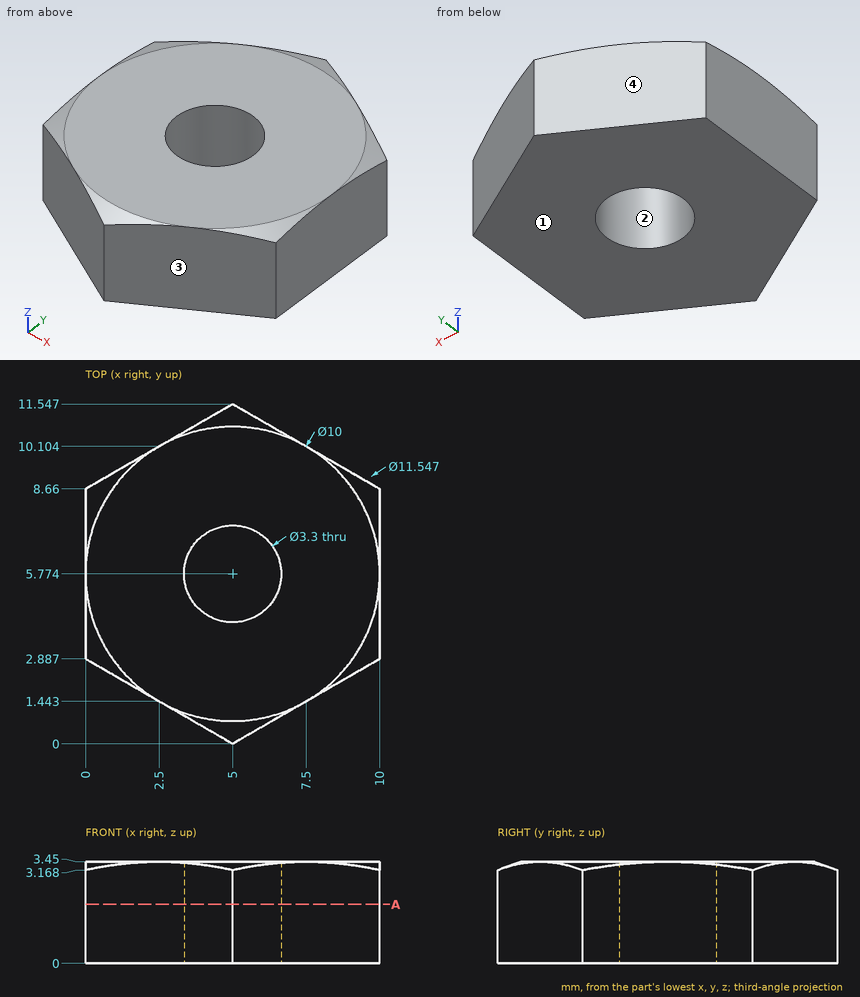
Design review of the part shown in the three views and the two pictorial views. Dimensions are in mm from the part's minimum x, y and z. Round coordinates to 2 decimals unless told otherwise and drop trailing zeros. Order: outer loops, then holes, each group sorted by start corner. A loop starts at its lowest first (then second) coordinate and runs counter-clockwise, first axis right, second up.
Item 1: To check wall thickness, follow probe 1 along X at (y, z) = (5.75, 2.5); probe 2 along X at (y, z) = (6.5, 1.1); probe 3 along Y at (x, z) = (4, 3.05) (1 decimal). State the ranges of each line that lie inside material, in increasing order.
Working result:
probe 1: x = 0 to 3.35, 6.65 to 10
probe 2: x = 0 to 3.52, 6.48 to 10
probe 3: y = 0.6 to 4.5, 7.1 to 11
Item 2: Add section A-A, the plane z = 2. State the section outline as (x, y) points.
Working result:
outline: (0, 2.89) - (5, 0) - (10, 2.89) - (10, 8.66) - (5, 11.55) - (0, 8.66) - close; hole circle Ø3.3 at (5, 5.77)
Item 3: Draft analysis for pull direction Y (two halves, no side actions). For the marked faces 1, 2, 3 and 4, state which applies: released by +Y, released by -Y, zero draft, split by the parting line, or undercut.
Working result:
face 1: zero draft
face 2: undercut
face 3: released by -Y
face 4: released by +Y
Item 4: For pin 1 (3 mm diameter, centred on x = 5, y = 5.77, fed in from +Z), flat-tipped, find the tip position at first contact; note if it passes through.
Working result:
pin 1: passes through
